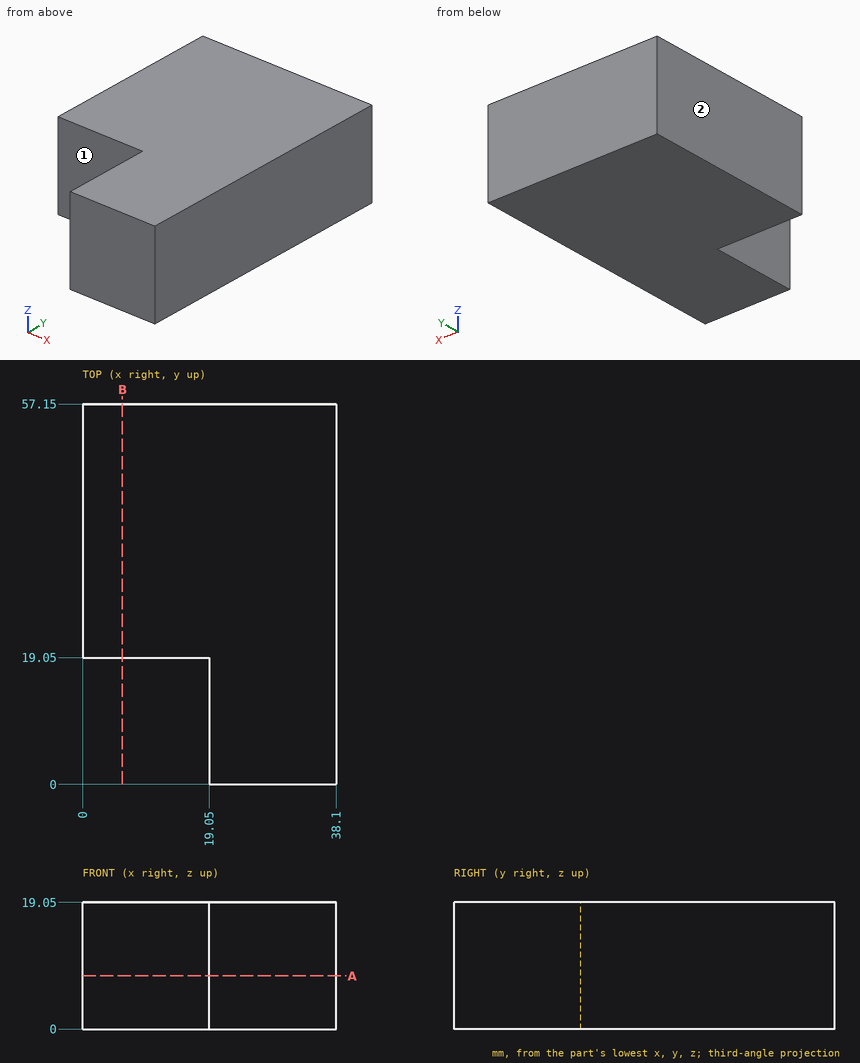
The drawing under review shows one solid part. Ordinate dimensions are in mm from its lowest x, y, z. A direction names the side the tool comes from. Round coordinates to 2 decimals unless told otherwise and drop trailing zeros. Order: outer loops, then holes, each group sorted by start corner. A loop starts at its lowest first (then second) coordinate and runs counter-clockwise, first axis right, second up. Notation, with made-up numbers: (25.5, 20.5) -> (81.5, 20.5) arc R24 cw to (81.5, 51.5) -> close; hole circle Ø2 at (75, -39). An arc over 180 degrees is marked (long way). Use a Markdown table: item, result.
Q1. Tool access review of the marked faces 1 and 2: name each direction out of +Z, -Z, +X, -X, +Y, -Y from which nothing blocks a thin tool from reaching the whole face with its end or side.
Values:
| item | result |
|---|---|
| face 1 | +Z, -Z, -X, -Y |
| face 2 | +Z, -Z, -X, +Y, -Y |
Q2. For line 1 (Y direction, x = 4.5, z = 10); line 2 (X direction, y = 11.5, z = 8.25), list the stretches that pass through material, from the lowest coordinate up.
Values:
| item | result |
|---|---|
| line 1 | y = 19.05 to 57.15 |
| line 2 | x = 19.05 to 38.1 |
Q3. We need section B-B on x = 6. Write out the cut boundary in (y, z).
Values:
| item | result |
|---|---|
| outline | (19.05, 0) -> (57.15, 0) -> (57.15, 19.05) -> (19.05, 19.05) -> close |
Q4. We need section A-A on z = 8. Write out the cut boundary in (x, y).
Values:
| item | result |
|---|---|
| outline | (0, 19.05) -> (19.05, 19.05) -> (19.05, 0) -> (38.1, 0) -> (38.1, 57.15) -> (0, 57.15) -> close |
Q5. Clearance check with a flat-ended pin moving along its axis: P1, Ø2, axis at y = 9.5, z = 16, coming from the -X side. State where the tip first meets the part, or that it passes through.
Values:
| item | result |
|---|---|
| P1 | stops at x = 19.05 |
